Here's the drawing with two shaded views (mm, measured from the low corner). I have some questions. Round coordinates to 2 decimals unless told otherwise and drop trailing zeros. Order: outer loops, then holes, each group sorted by start corner. A loop starts at its lowest first (then second) coordinate and runs counter-clockwise, first axis right, second up. Notation, with made-up numbers: (-6.5, 28) -> (0.5, 28) arc R25 ccw to (0.5, 64) -> close; hole circle Ø7 at (-19, 20). An arc over 180 degrees is marked (long way). Put each result on its own line as item: value. Start each with the question number.
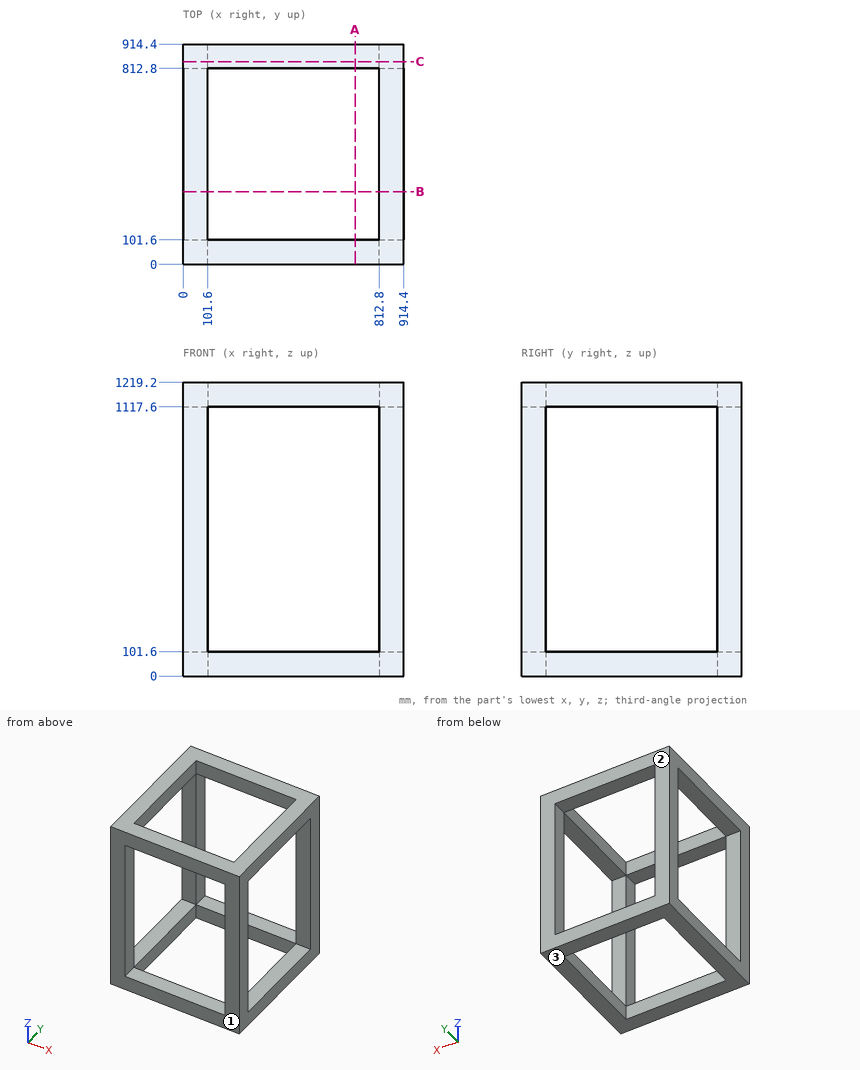
1. I need wall thicknesses on L1, parallel to X at y = 855.5, z = 1034; L2, parallel to Z at x = 829.5, y = 750. Which ranges of each line are inside material? Lowest first, please.
2. For pin 1 Ø8 at (y, z) = (806.5, 240.5) entering from -X, with a flat end and sliding along its axis, tell me the tip position at first contact or that it passes through.
3. If we section it at C-C, the plane y = 841: Please give me the cut outline in (x, z).
4. If we section it at A-A, the plane x = 713.5: Please give me the cut outline in (y, z).
5. Thinking about a two-plate mould opening in Y: for the marked faces 1, 2 and 3, which applies, +Y half, -Y half, draft (parallel to the pull), parting line (faces both ways), or undercut?
Results below:
1. L1: 0 to 101.6, 812.8 to 914.4
1. L2: 0 to 101.6, 1117.6 to 1219.2
2. pin 1: through
3. outline: (0, 0) -> (914.4, 0) -> (914.4, 1219.2) -> (0, 1219.2) -> close; hole (101.6, 101.6) -> (812.8, 101.6) -> (812.8, 1117.6) -> (101.6, 1117.6) -> close
4. outline: (0, 0) -> (101.6, 0) -> (101.6, 101.6) -> (0, 101.6) -> close; (0, 1117.6) -> (101.6, 1117.6) -> (101.6, 1219.2) -> (0, 1219.2) -> close; (812.8, 0) -> (914.4, 0) -> (914.4, 101.6) -> (812.8, 101.6) -> close; (812.8, 1117.6) -> (914.4, 1117.6) -> (914.4, 1219.2) -> (812.8, 1219.2) -> close
5. face 1: -Y half
5. face 2: +Y half
5. face 3: draft
